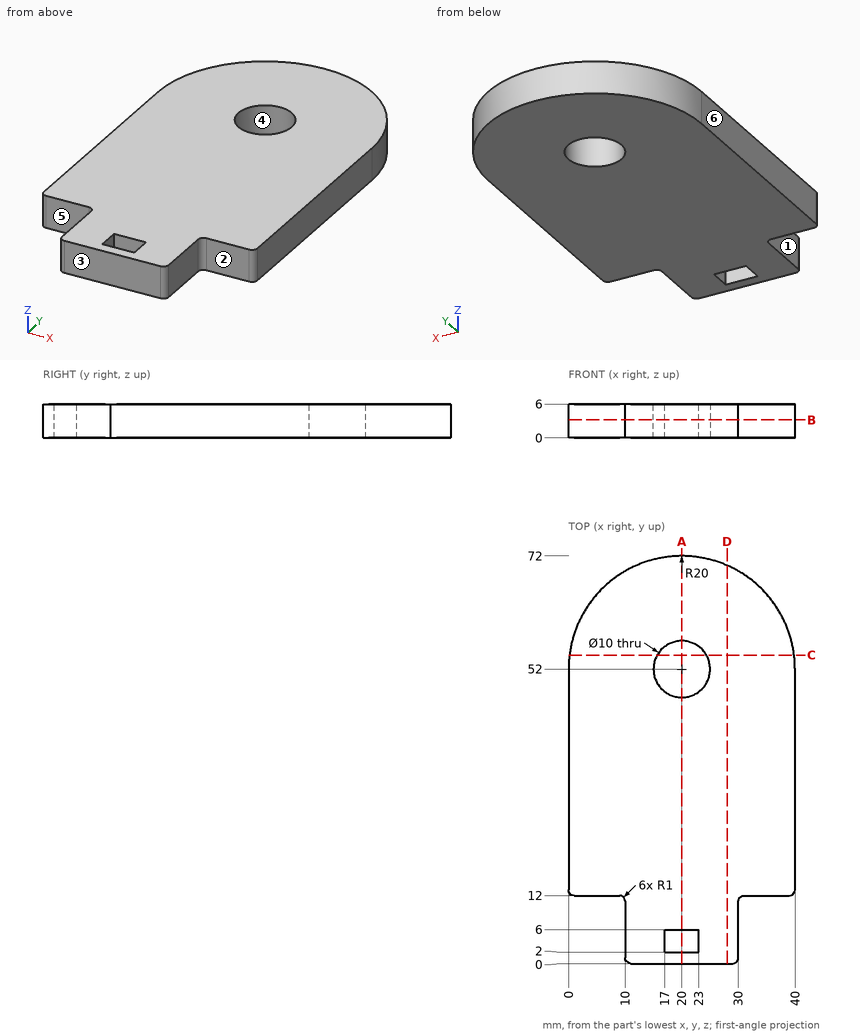
Design review of the part shown in the three views and the two pictorial views. Dimensions are in mm from the part's minimum x, y and z. A direction names the side the tool comes from. Round coordinates to 2 decimals unless told otherwise and drop trailing zeros. Write each loop counter-clockwise with the first axis right and the second up, starting at its lowest first coordinate (ties: lowest second). Pieces come first, ordered by that corner, then holes.
Item 1: Wall thickness on L1, parallel to Y at x = 20, z = 3.85; L2, parallel to Y at x = 22, z = 0.35; L3, parallel to X at y = 53, z = 0.85: over which ranges is each line inside the solid? List them lowest first.
Item 2: Consider section B-B on z = 3.2. Give the boundary of the cut face in (x, y).
Item 3: Consider section A-A on x = 20. Give the boundary of the cut face in (y, z).
Item 4: Consider section C-C on y = 54.5. Give the boundary of the cut face in (x, z), and give its area (3 significant figures).
Item 5: For the marked faces 1, 2 and 3, list the 3-axis set-ups (+Z, -Z, +X, -X, +Y, -Y) from which the entire face can be reached by the end or side of a thin tool; tool diameter is ignored.
Item 6: For pin 1 Ø1.8 at (x, z) = (5.5, 2.5) entering from -Y; pin 2 Ø3 at (y, z) = (7.5, 2) entering from -X; pin 3 Ø1.2 at (y, z) = (4, 4) entering from +X; pin 4 Ø6 at (x, y) = (20, 52) entering from +Z, all flat-tipped, find the tip position at first contact; note any pin that passes through.
Item 7: Draft analysis for pull direction X (two halves, no side actions). For the marked faces 4, 5 and 6, state which applies: released by +X, released by -X, zero draft, split by the parting line, or undercut.
Item 8: Consider section D-D on x = 28. Give the boundary of the cut face in (y, z).
Check values:
1. L1: y = 0 to 2, 6 to 47, 57 to 72
1. L2: y = 0 to 2, 6 to 47.42, 56.58 to 71.9
1. L3: x = 0.03 to 15.1, 24.9 to 39.97
2. outline: (0, 13) arc R1 ccw to (1, 12) - (9, 12) arc R1 cw to (10, 11) - (10, 1) arc R1 ccw to (11, 0) - (29, 0) arc R1 ccw to (30, 1) - (30, 11) arc R1 cw to (31, 12) - (39, 12) arc R1 ccw to (40, 13) - (40, 52) arc R20 ccw to (0, 52) - close; hole circle Ø10 at (20, 52); hole (17, 2) - (23, 2) - (23, 6) - (17, 6) - close
3. outline: (0, 0) - (2, 0) - (2, 6) - (0, 6) - close; (6, 0) - (47, 0) - (47, 6) - (6, 6) - close; (57, 0) - (72, 0) - (72, 6) - (57, 6) - close
4. outline: (0.16, 0) - (15.67, 0) - (15.67, 6) - (0.16, 6) - close; (24.33, 0) - (39.84, 0) - (39.84, 6) - (24.33, 6) - close
4. area: 186 mm2
5. face 1: +Z, -Z, -X, -Y
5. face 2: +Z, -Z, +X, -Y
5. face 3: +Z, -Z, +X, -X, -Y
6. pin 1: stops at y = 12
6. pin 2: stops at x = 10
6. pin 3: stops at x = 30
6. pin 4: passes through
7. face 4: undercut
7. face 5: zero draft
7. face 6: released by -X
8. outline: (0, 0) - (70.33, 0) - (70.33, 6) - (0, 6) - close
